from build123d import *

# Parameters (mm, degrees)
SKETCH1_R           = 2.54
SKETCH1_R_2         = 14.3002
BOSS_EXTRUDE1_DEPTH = 3.175


with BuildPart() as part:
    # Sketch1 → Boss-Extrude1 (new body)
    with BuildSketch(Plane(origin=(0, 0, 0), x_dir=(1, 0, 0), z_dir=(0, 1, 0))):
        with BuildLine():
            Line((0, 5.08), (0, 121.92))
            ThreePointArc((0, 121.92), (1.487897552, 125.512102448), (5.08, 127))
            Line((5.08, 127), (149.260387337, 127))
            ThreePointArc((149.260387337, 127), (151.931101387, 126.241306106), (153.804077467, 124.191845065))
            Line((153.804077467, 124.191845065), (202.66369013, 26.472619739))
            ThreePointArc((202.66369013, 26.472619739), (203.064104866, 25.367919511), (203.2, 24.200774674))
            Line((203.2, 24.200774674), (203.2, 5.08))
            ThreePointArc((203.2, 5.08), (201.712102448, 1.487897552), (198.12, 0))
            Line((198.12, 0), (5.08, 0))
            ThreePointArc((5.08, 0), (1.487897552, 1.487897552), (0, 5.08))
        make_face()
        with Locations(Location((190.5, 12.7, 0), (0, 0, 270))):
            Circle(SKETCH1_R, mode=Mode.SUBTRACT)
        with Locations(Location((165.1, 12.7, 0), (0, 0, 270))):
            Circle(SKETCH1_R, mode=Mode.SUBTRACT)
        with Locations(Location((139.7, 12.7, 0), (0, 0, 270))):
            Circle(SKETCH1_R, mode=Mode.SUBTRACT)
        with Locations(Location((114.3, 12.7, 0), (0, 0, 270))):
            Circle(SKETCH1_R, mode=Mode.SUBTRACT)
        with Locations(Location((88.9, 12.7, 0), (0, 0, 270))):
            Circle(SKETCH1_R, mode=Mode.SUBTRACT)
        with Locations(Location((63.5, 12.7, 0), (0, 0, 270))):
            Circle(SKETCH1_R, mode=Mode.SUBTRACT)
        with Locations(Location((38.1, 12.7, 0), (0, 0, 270))):
            Circle(SKETCH1_R, mode=Mode.SUBTRACT)
        with Locations(Location((12.7, 12.7, 0), (0, 0, 270))):
            Circle(SKETCH1_R, mode=Mode.SUBTRACT)
        with Locations(Location((12.7, 38.1, 0), (0, 0, 270))):
            Circle(SKETCH1_R, mode=Mode.SUBTRACT)
        with Locations(Location((139.7, 38.1, 0), (0, 0, 270))):
            Circle(SKETCH1_R, mode=Mode.SUBTRACT)
        with Locations(Location((12.7, 63.5, 0), (0, 0, 270))):
            Circle(SKETCH1_R, mode=Mode.SUBTRACT)
        with Locations(Location((139.7, 63.5, 0), (0, 0, 270))):
            Circle(SKETCH1_R, mode=Mode.SUBTRACT)
        with Locations(Location((12.7, 88.9, 0), (0, 0, 270))):
            Circle(SKETCH1_R, mode=Mode.SUBTRACT)
        with Locations(Location((139.7, 88.9, 0), (0, 0, 270))):
            Circle(SKETCH1_R, mode=Mode.SUBTRACT)
        with Locations(Location((12.7, 114.3, 0), (0, 0, 270))):
            Circle(SKETCH1_R, mode=Mode.SUBTRACT)
        with Locations(Location((139.7, 114.3, 0), (0, 0, 270))):
            Circle(SKETCH1_R, mode=Mode.SUBTRACT)
        with Locations(Location((63.5, 101.6, 0), (0, 0, 270))):
            Circle(SKETCH1_R_2, mode=Mode.SUBTRACT)
        with Locations(Location((63.5, 66.04, 0), (0, 0, 270))):
            Circle(SKETCH1_R_2, mode=Mode.SUBTRACT)
        with Locations(Location((91.360222469, 43.942, 0), (0, 0, 270))):
            Circle(SKETCH1_R_2, mode=Mode.SUBTRACT)
        with BuildLine():
            Line((93.98, 114.3), (121.92, 114.3))
            ThreePointArc((121.92, 114.3), (125.512102448, 112.812102448), (127, 109.22))
            Line((127, 109.22), (127, 68.58))
            ThreePointArc((127, 68.58), (125.512102448, 64.987897552), (121.92, 63.5))
            Line((121.92, 63.5), (93.98, 63.5))
            ThreePointArc((93.98, 63.5), (90.387897552, 64.987897552), (88.9, 68.58))
            Line((88.9, 68.58), (88.9, 109.22))
            ThreePointArc((88.9, 109.22), (90.387897552, 112.812102448), (93.98, 114.3))
        make_face(mode=Mode.SUBTRACT)
    extrude(amount=BOSS_EXTRUDE1_DEPTH)


solid = part.part
CAD build for the part. Positions are in the model's coordinates, mm. A direction names the side the tool comes from. Round coordinates to 2 decimals unless told otherwise and drop trailing zeros. Write each loop counter-clockwise with the first axis right and the second up, starting at its lowest first coordinate (ties: lowest second). Pieces come first, ordered by that corner, then holes. Notation, with made-up numbers: M -11,-38.75 L 34,-38.75 A16 cw 34,-12.75 Z; hole C -27.75,81.25 d2. An arc over 180 degrees is marked long. Put each result on its own line as item: value. Start each with the question number.
1) Pin check, flat tips, straight feed: pin 1 Ø1.5 at (y, z) = (1, -92) entering from +X (3 decimals); pin 2 Ø8 at (x, z) = (139.7, -12.7) entering from +Y (3 decimals). Stop position of each tip, or through.
2) Pull direction Z, two halves, no side cores. Call faces 1 (the flat face through (80, 3.175, -64)), 2 (the cylindrical face through (116.82, 1.57, -13.03)), 3 (the cylindrical face through (1.449, 1.565, -125.472)), 4 (the cylindrical face through (1.528, 1.565, -1.449)): pulls with the +Z half, pulls with the -Z half, needs draft (parallel to the pull), parting line crosses it, or undercut.
3) Saw through at A-A, the plane z = -101.6. Write the cut outline in (x, y) (3 decimals).
4) Saw through at C-C, the plane x = 59. Write the cut outline in (y, z) (3 decimals), and give its area (3 significant figures).
5) Saw through at B-B, the plane z = -38.1. Write the cut outline in (x, y) (3 decimals).
6) 3-axis set-ups, long thin cutter, end or side, ignore diameter. For faces 5 (the cylindrical face through (125.551, 1.565, -65.028)), 6 (the cylindrical face through (201.751, 1.565, -1.528)): which of +Z, -Z, +X, -X, +Y, -Y reach the whole face in a straight line?
7) Saw through at D-D, the plane x = 158. Write the cut outline in (y, z) (3 decimals).
8) Drill centre lines: probe 1 along Z at (x, y) = (139.7, 1.9); probe 2 along X at (y, z) = (2.25, -95); probe 3 along Z at (x, y) = (63, 1.75). Where is each one in solid material? Low to high. Write a range as [from, to].
Resolved:
1. pin 1: x = 170.275
1. pin 2: y = 3.175
2. face 1: needs draft
2. face 2: undercut
2. face 3: pulls with the -Z half
2. face 4: pulls with the +Z half
3. outline: M 0,0 L 49.2,0 L 49.2,3.175 L 0,3.175 Z; M 77.8,0 L 88.9,0 L 88.9,3.175 L 77.8,3.175 Z; M 127,0 L 165.1,0 L 165.1,3.175 L 127,3.175 Z
4. outline: M 0,-127 L 3.175,-127 L 3.175,-115.174 L 0,-115.174 Z; M 0,-88.026 L 3.175,-88.026 L 3.175,-79.614 L 0,-79.614 Z; M 0,-52.466 L 3.175,-52.466 L 3.175,0 L 0,0 Z
4. area: 231 mm²
5. outline: M 0,0 L 10.16,0 L 10.16,3.175 L 0,3.175 Z; M 15.24,0 L 78.308,0 L 78.308,3.175 L 15.24,3.175 Z; M 104.413,0 L 137.16,0 L 137.16,3.175 L 104.413,3.175 Z; M 142.24,0 L 196.85,0 L 196.85,3.175 L 142.24,3.175 Z
6. face 5: +Y, -Y
6. face 6: +Z, +X, +Y, -Y
7. outline: M 0,-115.8 L 3.175,-115.8 L 3.175,0 L 0,0 Z
8. probe 1: [-127, -116.84], [-111.76, -91.44], [-86.36, -66.04], [-60.96, -40.64], [-35.56, -15.24], [-10.16, 0]
8. probe 2: [0, 50.81], [76.19, 88.9], [127, 168.4]
8. probe 3: [-127, -115.89], [-87.31, -80.33], [-51.75, -15.19], [-10.21, 0]
